from build123d import *

# Parameters (mm, degrees)
SKETCH1_R           = 3.625
SKETCH1_R_2         = 2.075
BOSS_EXTRUDE1_DEPTH = 2.41
SKETCH2_R           = 1
SKETCH2_R_2         = 0.5
BOSS_EXTRUDE3_DEPTH = 1.89
BOSS_EXTRUDE4_START = 4.3
SKETCH1_2_R         = 3.625
SKETCH1_2_R_2       = 2.075
BOSS_EXTRUDE4_DEPTH = 0.8


with BuildPart() as part:
    # Sketch1 → Boss-Extrude1 (new body)
    with BuildSketch(Plane(origin=(0, 0, 0), x_dir=(1, 0, 0), z_dir=(0, 1, 0))):
        with Locations(Location((0, 0, 0), (0, 0, 270))):
            Circle(SKETCH1_R)
        with Locations(Location((0, 0, 0), (0, 0, 270))):
            Circle(SKETCH1_R_2, mode=Mode.SUBTRACT)
    extrude(amount=BOSS_EXTRUDE1_DEPTH)

    # Sketch2 → Boss-Extrude3 (add)
    with BuildSketch(Plane(origin=(0, 2.41, 0), x_dir=(1, 0, 0), z_dir=(0, 1, 0))):
        with BuildLine():
            Line((-10.6054557, -10.267177528), (-3.625, 0))
            ThreePointArc((-3.625, 0), (2.238819707, 2.851019347), (0.859585555, -3.521610097))
            Line((0.859585555, -3.521610097), (-7.459503317, -12.737599274))
            ThreePointArc((-7.459503317, -12.737599274), (-10.267690381, -13.075364593), (-10.6054557, -10.267177528))
        make_face()
        with Locations(Location((0, 0, 0), (0, 0, 270))):
            Circle(SKETCH2_R, mode=Mode.SUBTRACT)
        with Locations(Location((-9.032479508, -11.502388401, 0), (0, 0, 270))):
            Circle(SKETCH2_R_2, mode=Mode.SUBTRACT)
        with Locations(Location((-7.797268635, -9.92941221, 0), (0, 0, 270))):
            Circle(SKETCH2_R_2, mode=Mode.SUBTRACT)
        with Locations(Location((-6.562057762, -8.356436018, 0), (0, 0, 270))):
            Circle(SKETCH2_R_2, mode=Mode.SUBTRACT)
        with Locations(Location((-5.32684689, -6.783459826, 0), (0, 0, 270))):
            Circle(SKETCH2_R_2, mode=Mode.SUBTRACT)
        with Locations(Location((-4.091636017, -5.210483635, 0), (0, 0, 270))):
            Circle(SKETCH2_R_2, mode=Mode.SUBTRACT)
        with Locations(Location((-2.856425144, -3.637507443, 0), (0, 0, 270))):
            Circle(SKETCH2_R_2, mode=Mode.SUBTRACT)
    extrude(amount=BOSS_EXTRUDE3_DEPTH)

    # Sketch1<2> → Boss-Extrude4 (add)
    with BuildSketch(Plane(origin=(0, 0, 0), x_dir=(1, 0, 0), z_dir=(0, 1, 0)).offset(BOSS_EXTRUDE4_START)):
        with Locations(Location((0, 0, 0), (0, 0, 270))):
            Circle(SKETCH1_2_R)
        with Locations(Location((0, 0, 0), (0, 0, 270))):
            Circle(SKETCH1_2_R_2, mode=Mode.SUBTRACT)
    extrude(amount=BOSS_EXTRUDE4_DEPTH)


solid = part.part
Geometry check sheet. Reference: the model listing, model coordinates, mm. A direction names the side the tool comes from. Give positions to 0.01 mm unless a question says otherwise; leave off trailing zeros. Order: outer loops, then holes, each group sorted by start corner. A loop starts at its lowest first (then second) coordinate and runs counter-clockwise, first axis right, second up. Notation, with made-up numbers: (71, 29.5) - (129, 29.5) arc R14 ccw to (129, 52.5) - close; hole circle Ø5 at (83, 31.25). An arc over 180 degrees is marked (long way). Answer as a JSON object with one key per item and string values.
(1) Tool access check on faces 5 (the cylindrical face through (-1.26, 4.69, -1.65)), 6 (the cylindrical face through (-2.83, 3.34, 3.14)). Record the directions out of +Z, -Z, +X, -X, +Y, -Y that give a thin tool (end or side, any length) a straight path to the whole face; none if there is none.
Report:
{"face 5": "+Y", "face 6": "+Y, -Y"}
(2) Depth check by flat-ended pin: pin 1 Ø1.5 at (y, z) = (4.5, 10.5) entering from +X; pin 2 Ø1 at (y, z) = (4.5, 3.5) entering from +X; pin 3 Ø6 at (x, z) = (-4.5, 5) entering from +Y. Enter the tip coordinate at first touch or a pass-through.
Report:
{"pin 1": "x = -4.79", "pin 2": "x = 2.03", "pin 3": "y = 4.3"}
(3) Draft check along X on faces 1 (the cylindrical face through (-10.233, 3.342, 13.102)), 2 (the flat face through (-3.242, 3.342, 8.065)), 3 (the cylindrical face through (-1.26, 1.19, -1.65)), 4 (the flat face through (-6, 2.41, 7)). Enter one of: released by +X, released by -X, zero draft, split by the parting line, or undercut.
Report:
{"face 1": "split by the parting line", "face 2": "released by +X", "face 3": "undercut", "face 4": "zero draft"}
(4) Cross-section at D-D (z = 12.25). Record the cut outline in (x, y), then the cut area to 3 significant figures.
Report:
{"outline": "(-10.89, 2.41) - (-7.02, 2.41) - (-7.02, 4.3) - (-10.89, 4.3) - close", "area": "7.31 mm^2"}
(5) Cross-section at B-B (y = 4.1). State how many separate pieces and enclosed holes the cut face has, then the cut area to 3 significant figures.
Report:
{"separate pieces": "1", "enclosed holes": "7", "area": "94.3 mm^2"}
(6) Cross-section at C-C (x = -0.5). Record the cut outline in (y, z).
Report:
{"outline": "(0, -3.59) - (5.1, -3.59) - (5.1, -2.01) - (4.3, -2.01) - (4.3, -0.87) - (2.41, -0.87) - (2.41, -2.01) - (0, -2.01) - close; (0, 2.01) - (2.41, 2.01) - (2.41, 0.87) - (4.3, 0.87) - (4.3, 2.01) - (5.1, 2.01) - (5.1, 3.59) - (4.3, 3.59) - (4.3, 5.03) - (2.41, 5.03) - (2.41, 3.59) - (0, 3.59) - close"}
(7) Cross-section at A-A (x = -8). Record the cut outline in (y, z), then the cut area to 3 significant figures.
Report:
{"outline": "(2.41, 6.43) - (4.3, 6.43) - (4.3, 9.47) - (2.41, 9.47) - close; (2.41, 10.39) - (4.3, 10.39) - (4.3, 13.22) - (2.41, 13.22) - close", "area": "11.1 mm^2"}
(8) Material ranges on line 1 (X direction, y = 4.9, z = 0) (3 decimals); line 2 (X direction, y = 3.4, z = 0) (3 decimals); line 3 (Z direction, x = 1.5, y = 2.05), recorded low to high.
Report:
{"line 1": "-3.625 to -2.075, 2.075 to 3.625", "line 2": "-3.625 to -1, 1 to 3.625", "line 3": "-3.3 to -1.43, 1.43 to 3.3"}
